Part model, mm, in its own coordinate system. Give positions to 0.01 mm unless a question says otherwise; leave off trailing zeros. Write each loop counter-clockwise with the first axis right and the second up, starting at its lowest first coordinate (ties: lowest second). Pieces come first, ordered by that corner, then holes. Notation, with made-up numbers: (1.25, 66.25) - (16.25, 66.25) arc R12 cw to (16.25, 76.25) - close; hole circle Ø2 at (-37, -24.5). An arc over 180 degrees is marked (long way). Answer in a Markdown table with one row per item. Add a question column.
1. Band-saw the part on C-C on y = 1.3. Write the cut outline in (x, z), plus the area to 3 significant figures.
2. Band-saw the part on A-A on z = 0. Write the cut outline in (x, y), plus the area to 3 significant figures.
3. Band-saw the part on B-B on y = 4.05. Write the cut outline in (x, z), plus the area to 3 significant figures.
4. Drop flat-ended pins along their axis: pin 1 Ø2 at (x, y) = (-21.5, 0.5) entering from -Z; pin 2 Ø2.5 at (x, z) = (-10.5, 0) entering from +Y; pin 3 Ø2 at (y, z) = (1, -3.5) entering from -X; pin 4 Ø1 at (x, y) = (-21.5, 0.5) entering from -Z (3 decimals). Give the stop position or say it passes through.
5. Probe line 1 along X through (y, z) = (1.7, 1); line 2 along Z through (x, y) = (-11.5, 2.7); line 3 along Z through (x, y) = (-20.5, 3.4). List the from-to ranges inside material, lowest first.
```python
from build123d import *

# Parameters (mm, degrees)
BOSS_EXTRUDE2_DEPTH       = 5
F_4_0MM_DOWEL_HOLE1_D     = 4
F_4_0MM_DOWEL_HOLE1_DEPTH = 117.6291
F_4_0MM_DOWEL_HOLE1_TIP   = 1.201721238
FILLET1_R                 = 2


with BuildPart() as part:
    # Sketch2 → Boss-Extrude2 (new body)
    with BuildSketch(Plane(origin=(0, 0, 0), x_dir=(1, 0, 0), z_dir=(0, 1, 0))):
        with BuildLine():
            Line((-5, 30.087372767), (-5, -30.087372767))
            ThreePointArc((-5, -30.087372767), (-30.5, 0), (-5, 30.087372767))
        make_face()
    extrude(amount=BOSS_EXTRUDE2_DEPTH)

    # Ø4.0mm Dowel Hole1
    with Locations(Plane.XZ):
        with Locations((-20.5, 0), (-10.5, 0)):
            Hole(F_4_0MM_DOWEL_HOLE1_D / 2, depth=F_4_0MM_DOWEL_HOLE1_DEPTH)
            with Locations((0, 0, -(F_4_0MM_DOWEL_HOLE1_DEPTH + F_4_0MM_DOWEL_HOLE1_TIP / 2))):  # 118° drill point
                Cone(0, F_4_0MM_DOWEL_HOLE1_D / 2, F_4_0MM_DOWEL_HOLE1_TIP, mode=Mode.SUBTRACT)

    # Fillet1
    fillet1_edges = [part.edges().sort_by_distance(p)[0] for p in [
        (-5, 0, 0),
        (-30.5, 0, 0),
        (-5, 2.5, -30.087372767),
        (-5, 2.5, 30.087372767),
    ]]
    fillet(fillet1_edges, radius=FILLET1_R)


solid = part.part
```
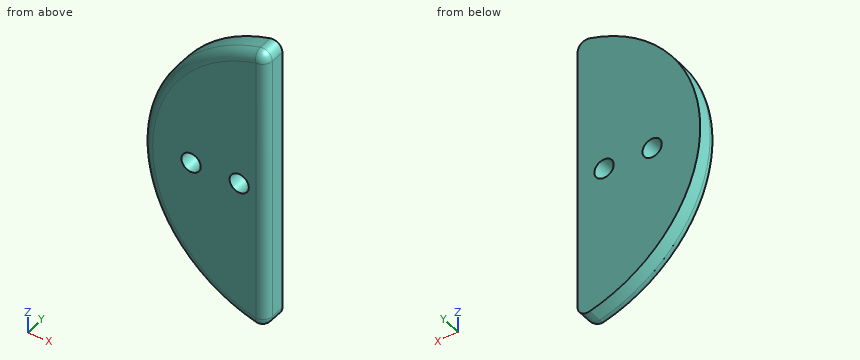
Values:
| question | item | result |
|---|---|---|
| 1 | outline | (-7.46, -29.44) arc R1.87 ccw to (-5.13, -27.63) - (-5.13, 27.63) arc R1.87 ccw to (-7.46, 29.44) arc R30.37 ccw to start; hole circle Ø4 at (-20.5, 0); hole circle Ø4 at (-10.5, 0) |
| 1 | area | 1,110 mm² |
| 2 | outline | (-30.5, 2) arc R2 ccw to (-28.5, 0) - (-22.5, 0) - (-22.5, 5) - (-30.5, 5) - close; (-18.5, 0) - (-12.5, 0) - (-12.5, 5) - (-18.5, 5) - close; (-8.5, 0) - (-7, 0) arc R2 ccw to (-5, 2) - (-5, 5) - (-8.5, 5) - close |
| 2 | area | 85.8 mm² |
| 3 | outline | (-7.49, -29.57) arc R2 ccw to (-5, -27.63) - (-5, 27.63) arc R2 ccw to (-7.49, 29.57) arc R30.5 ccw to start; hole circle Ø4 at (-20.5, 0); hole circle Ø4 at (-10.5, 0) |
| 3 | area | 1,130 mm² |
| 4 | pin 1 | stops at z = -22.11 |
| 4 | pin 2 | passes through |
| 4 | pin 3 | stops at x = -30.35 |
| 4 | pin 4 | stops at z = -21.475 |
| 5 | line 1 | x = -30.46 to -22.23, -18.77 to -12.23, -8.77 to -5.02 |
| 5 | line 2 | z = -28.25 to -1.73, 1.73 to 28.25 |
| 5 | line 3 | z = -22.58 to -2, 2 to 22.58 |
